from build123d import *

# Parameters (mm, degrees)
SKETCH1_W           = 160
SKETCH1_H           = 160
BOSS_EXTRUDE1_DEPTH = 4
SKETCH2_W           = 4
SKETCH2_H           = 25
SKETCH2_H_2         = 10
CUT_EXTRUDE1_DEPTH  = 5
CIRPATTERN1_COUNT   = 4


with BuildPart() as part:
    # Sketch1 → Boss-Extrude1 (new body)
    with BuildSketch(Plane(origin=(0, 0, 0), x_dir=(1, 0, 0), z_dir=(0, 1, 0))):
        Rectangle(SKETCH1_W, SKETCH1_H)
    extrude(amount=BOSS_EXTRUDE1_DEPTH)

    # Sketch2 → Cut-Extrude1 (cut, through all)
    with BuildSketch(Plane(origin=(0, 4, 0), x_dir=(1, 0, 0), z_dir=(0, 1, 0))):
        with Locations((0, -12.5)):
            Rectangle(SKETCH2_W, SKETCH2_H)
        with Locations((0, -40)):
            Rectangle(SKETCH2_W, SKETCH2_H_2)
        with Locations((0, -60)):
            Rectangle(SKETCH2_W, SKETCH2_H_2)
    cut_extrude1 = extrude(amount=-CUT_EXTRUDE1_DEPTH, mode=Mode.SUBTRACT)

    # CirPattern1: Cut-Extrude1 ×4 about axis
    cirpattern1_axis = Axis((0, 0, 0), (0, 1, 0))
    for i in range(1, CIRPATTERN1_COUNT):
        add(cut_extrude1.rotate(cirpattern1_axis, i * 360 / CIRPATTERN1_COUNT), mode=Mode.SUBTRACT)


solid = part.part
For this review, take the finished solid that the model builds, in its own axes (mm). A direction names the side the tool comes from. Round coordinates to 2 decimals unless told otherwise and drop trailing zeros. Order: outer loops, then holes, each group sorted by start corner. A loop starts at its lowest first (then second) coordinate and runs counter-clockwise, first axis right, second up. Notation, with made-up numbers: (-16, 55) -> (5, 55) arc R21 cw to (5, 81) -> close; hole circle Ø4 at (7.5, 3.25). An arc over 180 degrees is marked (long way). Write item = value, one per line. Start each with the question number.
1) Take a section at A-A on x = -58.5. State the section outline as (y, z) points.
2) Take a section at C-C on y = 2.45. Count the separate pieces of the cut face and the enclosed holes in it, plus the area to 3 significant figures.
3) Take a section at B-B on z = -62.5. State the section outline as (x, y) points, plus the area to 3 significant figures.
4) Tool access review of faces 1 (the face through (-55, 2, 0)), 2 (the face through (17, 0, 17)): name each direction out of +Z, -Z, +X, -X, +Y, -Y from which nothing blocks a thin tool from reaching the whole face with its end or side.
5) The part is to be moulded in two halves that separate along Z. For faces 3 (the face through (80, 2, 1)), 4 (the face through (-2, 2, -14)), 5 (the face through (0, 2, -45)), say which applies: +Z half, -Z half, draft (parallel to the pull), parting line (faces both ways), or undercut.
6) To check wall thickness, follow line 1 (X direction, y = 1.6, z = 38); line 2 (X direction, y = 0.85, z = -1.5). State the ranges of each line that lie inside material, in increasing order. Write a range as from..to.
Verdict:
q1.outline = (0, -80) -> (4, -80) -> (4, -2) -> (0, -2) -> close; (0, 2) -> (4, 2) -> (4, 80) -> (0, 80) -> close
q2.separate_pieces = 1
q2.enclosed_holes = 9
q2.area = 24,900 mm2
q3.outline = (-80, 0) -> (-2, 0) -> (-2, 4) -> (-80, 4) -> close; (2, 0) -> (80, 0) -> (80, 4) -> (2, 4) -> close
q3.area = 624 mm2
q4.face_1 = +Y, -Y
q4.face_2 = +Z, -Z, +X, -X, -Y
q5.face_3 = draft
q5.face_4 = undercut
q5.face_5 = undercut
q6.line_1 = -80..-2, 2..80
q6.line_2 = -80..-65, -55..-45, -35..-25, 25..35, 45..55, 65..80
